For this review, take the finished solid that the model builds, in its own axes (mm). Give positions to 0.01 mm unless a question says otherwise; leave off trailing zeros. Order: outer loops, then holes, each group sorted by start corner. A loop starts at its lowest first (then second) coordinate and runs counter-clockwise, first axis right, second up. Notation, with made-up numbers: M 85.25,89 L 123.25,89 A29 cw 123.25,110 Z; hole C 50,46.25 d4. An arc over 180 degrees is marked long. Use CSV: the item, a comma, the result in double quotes. Start each with the question number.
(1) Consider section C-C (x = 63). Write out the cut boundary in (y, z).
(2) Draft analysis for pull direction Z (two halves, no side actions). For faces 1 (the face through (42.45, 23.1, -1.97)), 2 (the face through (0, 5.3, 0)), 3 (the face through (-2.436, 2.613, -1.868)), 4 (the face through (0, 31.55, 0)), state which applies: pulls with the +Z half, pulls with the -Z half, needs draft (parallel to the pull), parting line crosses it, or undercut.
(3) Clearance check with flat-ended pins moving along their axes: P1, Ø4, axis at y = 4.5, z = 1, coming from the +X side; P2, Ø12, axis at x = 20, y = 26, coming from the +Z side; P3, Ø5, axis at x = 29.5, z = -2.5, coming from the +Y side; P4, Ø1.5, axis at x = 6.5, y = 19, coming from the +Z side. State where each tip first meets the part, or that it passes through.
(4) Wall thickness on L1, parallel to Z at x = 0, y = 2; L2, parallel to Y at x = 50, z = -0.5; L3, parallel to Y at x = 70.5, z = -3: over which ranges is each line inside the solid? List them lowest first. Write a range as from..to.
(5) Consider section B-B (y = 21). Write out the cut boundary in (x, z), and give its area (3 significant figures).
(6) Consider section A-A (x = 0). Write out the cut boundary in (y, z).
```python
from build123d import *

# Parameters (mm, degrees)
SKETCH1_R           = 4.95
BOSS_EXTRUDE1_DEPTH = 31.55
SKETCH3_R           = 4.65
BOSS_EXTRUDE2_DEPTH = 85.9
BOSS_EXTRUDE2_TAPER = 0.5
FILLET1_R           = 3.9
SKETCH4_R           = 3.07
CUT_EXTRUDE1_DEPTH  = 5.3


with BuildPart() as part:
    # Sketch1 → Boss-Extrude1 (new body)
    with BuildSketch(Plane(origin=(0, 0, 0), x_dir=(1, 0, 0), z_dir=(0, 1, 0))):
        Circle(SKETCH1_R)
    extrude(amount=BOSS_EXTRUDE1_DEPTH)

    # Sketch3 → Boss-Extrude2 (add)
    with BuildSketch(Plane(origin=(0, 0, 0), x_dir=(0, 0, -1), z_dir=(1, 0, 0))):
        with Locations((0, 26.9)):
            Circle(SKETCH3_R)
    extrude(amount=BOSS_EXTRUDE2_DEPTH, taper=BOSS_EXTRUDE2_TAPER)

    # Fillet1
    fillet1_edges = [part.edges().sort_by_distance(p)[0] for p in [
        (85.9, 26.9, 3.900362057),
    ]]
    fillet(fillet1_edges, radius=FILLET1_R)

    # Sketch4 → Cut-Extrude1 (cut)
    with BuildSketch(Plane.XZ):
        Circle(SKETCH4_R)
    extrude(amount=-CUT_EXTRUDE1_DEPTH, mode=Mode.SUBTRACT)


solid = part.part
```
Check result:
1,outline,"C 26.9,0 d8.2"
2,face 1,"parting line crosses it"
2,face 2,"undercut"
2,face 3,"undercut"
2,face 4,"needs draft"
3,P1,"stops at x = 4.95"
3,P2,"stops at z = 4.53"
3,P3,"stops at y = 31.3"
3,P4,"passes through"
4,L1,"z = -4.95..-3.07, 3.07..4.95"
4,L2,"y = 22.72..31.08"
4,L3,"y = 24.2..29.6"
5,outline,"C 0,0 d9.9"
5,area,"77.0 mm^2"
6,outline,"M 0,-4.95 L 31.55,-4.95 L 31.55,4.95 L 0,4.95 L 0,3.07 L 5.3,3.07 L 5.3,-3.07 L 0,-3.07 Z"
